Read the model definition and answer for the solid it produces. Units are mm, in the model's axes. A direction names the side the tool comes from. Coordinates: 2 decimals unless noted, no trailing zeros. Order: outer loops, then holes, each group sorted by start corner. A loop starts at its lowest first (then second) coordinate and runs counter-clockwise, first axis right, second up. Notation, with made-up numbers: M 8.25,-18.5 L 43.25,-18.5 A28 cw 43.25,8.5 Z; hole C -14,34 d8. An arc over 180 degrees is marked long. Use a Markdown table: item, result. Add a question column.
1) Find section D-D on y = 0.9. Write down the section's boundary in (x, z).
2) Find the intervals of material crossed by probe 1 along Z at (x, y) = (-25, 2.6); probe 2 along Z at (x, y) = (-46, 1.9); probe 3 along Z at (x, y) = (-35, 1.2), in increasing order. Write a range as [from, to].
3) Find section A-A on z = -12. Write down the section's boundary in (x, y), plus the area to 3 significant figures.
4) Each of these flat-tipped pins is pushed along its axis until it touches: pin 1 Ø1.6 at (x, z) = (-25.5, -30) entering from -Y; pin 2 Ø1 at (x, z) = (-45.5, -0.5) entering from -Y. Where does it stop, or does it pass through?
5) For faces 4 (the face through (-25, 2.8, 0)), 5 (the face through (-48.54, 1.52, 4.95)), determine the directions among +Z, -Z, +X, -X, +Y, -Y from which every point of the face is accessible in a straight line to the end or side of a thin tool.
6) The mould has two halves that part along Z. Classify faces 1 (the face through (-36, 1, 5.804)), 2 (the face through (-31, 3, -16)), 3 (the face through (-43.59, 1.38, 0.87)): released by +Z, released by -Z, zero draft, split by the parting line, or undercut.
7) Find section B-B on x = -38.5. Write down the section's boundary in (y, z).
8) Find section C-C on x = -24. Write down the section's boundary in (y, z).
from build123d import *

# Parameters (mm, degrees)
SZKIC1_R                        = 1.65
SZKIC1_R_2                      = 7.798887489
DODANIE_WYCI_GNI_CIE1_DEPTH     = 3
ZAOKR_GLENIE1_R                 = 5
WYTNIJ_WYCI_GNI_CIE1_DEPTH      = 72.750306382
WYTNIJ_WYCI_GNI_CIE1_DEPTH_BACK = 72.750306382
SZKIC2_W                        = 22.67550991
SZKIC2_H                        = 46.936854919
ZAOKR_GLENIE5_R                 = 3
SZKIC3_R                        = 1.65
WYTNIJ_WYCI_GNI_CIE2_DEPTH      = 62.58622378
DODANIE_WYCI_GNI_CIE2_START     = -0.2
SZKIC4_R                        = 1.65
DODANIE_WYCI_GNI_CIE2_DEPTH     = 0.2


with BuildPart() as part:
    # Szkic1 → Dodanie-wyciągnięcie1 (new body)
    with BuildSketch(Plane(origin=(0, 0, 0), x_dir=(1, 0, 0), z_dir=(0, 1, 0))):
        with BuildLine():
            ThreePointArc((-57.522805166, 36.596117071), (-60.573917858, 31.893472489), (-61.642766658, 26.390589884))
            Line((-61.642766658, 26.390589884), (-61.642766658, 4.401644259))
            ThreePointArc((-61.642766658, 4.401644259), (-60.573917858, -1.101238346), (-57.522805166, -5.803882929))
            Line((-57.522805166, -5.803882929), (-23.176157761, -5.803882929))
            Line((-23.176157761, -5.803882929), (-19.042766658, -1.670491825))
            Line((-19.042766658, -1.670491825), (-19.042766658, 32.462725968))
            Line((-19.042766658, 32.462725968), (-23.176157761, 36.596117071))
            Line((-23.176157761, 36.596117071), (-57.522805166, 36.596117071))
        make_face()
        with Locations(Location((-55.942766658, -0.103882929, 0), (0, 0, 270))):
            Circle(SZKIC1_R, mode=Mode.SUBTRACT)
        with Locations(Location((-24.942766658, -0.103882929, 0), (0, 0, 270))):
            Circle(SZKIC1_R, mode=Mode.SUBTRACT)
        with Locations(Location((-55.942766658, 30.896117071, 0), (0, 0, 270))):
            Circle(SZKIC1_R, mode=Mode.SUBTRACT)
        with Locations(Location((-24.942766658, 30.896117071, 0), (0, 0, 270))):
            Circle(SZKIC1_R, mode=Mode.SUBTRACT)
        with Locations(Location((-40.442766658, 15.396117071, 0), (0, 0, 270))):
            Circle(SZKIC1_R_2, mode=Mode.SUBTRACT)
    extrude(amount=DODANIE_WYCI_GNI_CIE1_DEPTH)

    # Zaokrąglenie1
    zaokr_glenie1_edges = [part.edges().sort_by_distance(p)[0] for p in [
        (-23.176157761, 1.5, -36.596117071),
        (-19.042766658, 1.5, -32.462725968),
        (-19.042766658, 1.5, 1.670491825),
        (-23.176157761, 1.5, 5.803882929),
        (-57.522805166, 1.5, 5.803882929),
        (-57.522805166, 1.5, -36.596117071),
    ]]
    fillet(zaokr_glenie1_edges, radius=ZAOKR_GLENIE1_R)

    # Szkic2 → Wytnij-wyciągnięcie1 (cut, two sides: drawn at the far end of the back side and taken through both)
    with BuildSketch(Plane.XZ.offset(-WYTNIJ_WYCI_GNI_CIE1_DEPTH_BACK)):
        with Locations((-60.780521613, -15.396117072)):
            Rectangle(SZKIC2_W, SZKIC2_H)
    extrude(amount=WYTNIJ_WYCI_GNI_CIE1_DEPTH + WYTNIJ_WYCI_GNI_CIE1_DEPTH_BACK, mode=Mode.SUBTRACT)

    # Zaokrąglenie5
    zaokr_glenie5_edges = [part.edges().sort_by_distance(p)[0] for p in [
        (-49.442766658, 1.5, -36.596117071),
        (-49.442766658, 1.5, 5.803882929),
    ]]
    fillet(zaokr_glenie5_edges, radius=ZAOKR_GLENIE5_R)

    # Szkic3 → Wytnij-wyciągnięcie2 (cut, through all)
    with BuildSketch(Plane.XZ):
        with Locations(Location((-45.052026831, -30.896117071, 0), (0, 0, 90))):
            Circle(SZKIC3_R)
        with Locations(Location((-45.052026831, 0.103882929, 0), (0, 0, 90))):
            Circle(SZKIC3_R)
    extrude(amount=-WYTNIJ_WYCI_GNI_CIE2_DEPTH, mode=Mode.SUBTRACT)

    # Szkic4 → Dodanie-wyciągnięcie2 (add)
    with BuildSketch(Plane(origin=(0, 3, 0), x_dir=(1, 0, 0), z_dir=(0, 1, 0)).offset(DODANIE_WYCI_GNI_CIE2_START)):
        with Locations(Location((-45.052026831, 30.896117071, 0), (0, 0, 270))):
            Circle(SZKIC4_R)
        with Locations(Location((-24.942766658, 30.896117071, 0), (0, 0, 270))):
            Circle(SZKIC4_R)
        with Locations(Location((-24.942766658, -0.103882929, 0), (0, 0, 270))):
            Circle(SZKIC4_R)
        with Locations(Location((-45.052026831, -0.103882929, 0), (0, 0, 270))):
            Circle(SZKIC4_R)
    extrude(amount=DODANIE_WYCI_GNI_CIE2_DEPTH)


solid = part.part
Check result:
| question | item | result |
|---|---|---|
| 1 | outline | M -49.44,-33.6 A3 ccw -46.44,-36.6 L -25.25,-36.6 A5 ccw -21.71,-35.13 L -20.51,-33.93 A5 ccw -19.04,-30.39 L -19.04,-0.4 A5 ccw -20.51,3.13 L -21.71,4.34 A5 ccw -25.25,5.8 L -46.44,5.8 A3 ccw -49.44,2.8 Z; hole C -40.44,-15.4 d15.6; hole C -45.05,-30.9 d3.3; hole C -45.05,0.1 d3.3; hole C -24.94,-30.9 d3.3; hole C -24.94,0.1 d3.3 |
| 2 | probe 1 | z = [-36.59, -32.55], [-29.25, -1.55], [1.75, 5.8] |
| 2 | probe 2 | z = [-36.6, -32.25], [-29.55, -20.87], [-9.92, -1.25], [1.45, 5.8] |
| 2 | probe 3 | z = [-36.6, -20.98], [-9.81, 5.8] |
| 3 | outline | M -49.44,0 L -47.46,0 L -47.46,3 L -49.44,3 Z; M -33.42,0 L -19.04,0 L -19.04,3 L -33.42,3 Z |
| 3 | area | 49.1 mm2 |
| 4 | pin 1 | stops at y = 0 |
| 4 | pin 2 | stops at y = 2.8 |
| 5 | face 4 | -Y |
| 5 | face 5 | +Z, -X, +Y, -Y |
| 6 | face 1 | released by +Z |
| 6 | face 2 | zero draft |
| 6 | face 3 | undercut |
| 7 | outline | M 0,-36.6 L 3,-36.6 L 3,-22.95 L 0,-22.95 Z; M 0,-7.84 L 3,-7.84 L 3,5.8 L 0,5.8 Z |
| 8 | outline | M 0,-36.44 L 3,-36.44 L 3,5.65 L 0,5.65 L 0,1.46 L 2.8,1.46 L 2.8,-1.25 L 0,-1.25 L 0,-29.54 L 2.8,-29.54 L 2.8,-32.25 L 0,-32.25 Z |
